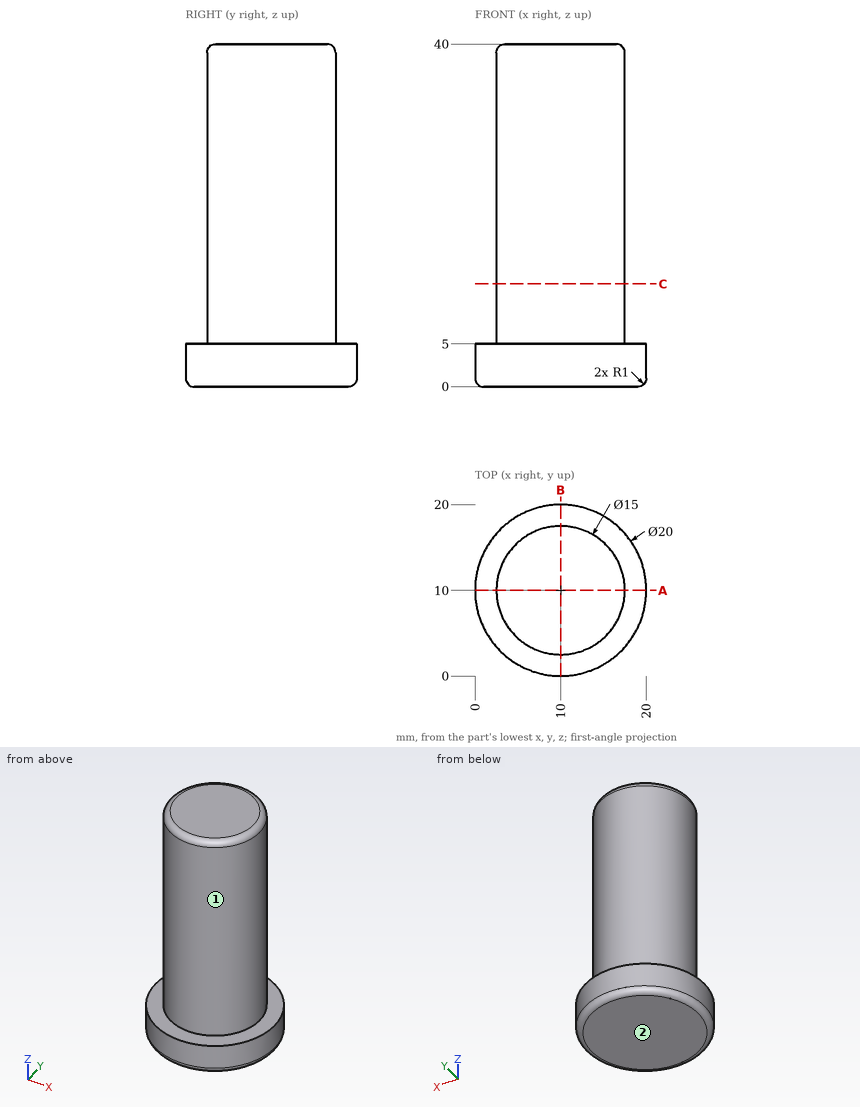
Drawing for the job (mm, zero at the part's lowest x, y, z). A direction names the side the tool comes from. Coordinates: 2 decimals unless noted, no trailing zeros. Order: outer loops, then holes, each group sorted by start corner. A loop starts at its lowest first (then second) coordinate and runs counter-clockwise, first axis right, second up. Notation, with made-up numbers: (83, 59) -> (91, 59) arc R27 ccw to (91, 94) -> close; hole circle Ø10 at (55, -30). An arc over 180 degrees is marked (long way). Answer in a Markdown table with one row per item.
1) Drill centre lines: line 1 (Z direction, x = 7, y = 2); line 2 (X direction, y = 10.5, z = 2); line 3 (Y direction, x = 16.5, z = 26). Where is each one in solid material? Low to high.
Check values:
| item | result |
|---|---|
| line 1 | 0 to 5 |
| line 2 | 0.01 to 19.99 |
| line 3 | 6.26 to 13.74 |
2) Band-saw the part on C-C (z = 12). List the corners of the cut face in (x, y).
Check values:
| item | result |
|---|---|
| outline | circle Ø15 at (10, 10) |
3) Band-saw the part on A-A (y = 10). List the corners of the cut face in (x, z).
Check values:
| item | result |
|---|---|
| outline | (0, 1) arc R1 ccw to (1, 0) -> (19, 0) arc R1 ccw to (20, 1) -> (20, 5) -> (17.5, 5) -> (17.5, 39) arc R1 ccw to (16.5, 40) -> (3.5, 40) arc R1 ccw to (2.5, 39) -> (2.5, 5) -> (0, 5) -> close |
4) Flat gauge pins, fed straight in: P1, Ø2, axis at x = 5, z = 31.5, coming from the -Y side; P2, Ø2, axis at y = 9.5, z = 6.5, coming from the +X side; P3, Ø10, axis at x = 8, z = 35.5, coming from the -Y side. Where does each tip first touch, or does it go through?
Check values:
| item | result |
|---|---|
| P1 | y = 3.66 |
| P2 | x = 17.5 |
| P3 | y = 2.5 |
5) Which spindle directions (+Z, -Z, +X, -X, +Y, -Y) get a long thin tool onto all of the face, cutting with end or side? Do the marked faces 1 and 2. Say none if no direction does.
Check values:
| item | result |
|---|---|
| face 1 | +Z |
| face 2 | -Z, +X, -X, +Y, -Y |
